Input: part model. Units: mm. Frame: model coordinates. A direction names the side the tool comes from. Give positions to 0.01 mm unless a question says otherwise; leave off trailing zeros. Loops run counter-clockwise (first coordinate to the right, second up) from the corner with the lowest first, then second, coordinate; pieces in that order, holes last. Notation, with made-up numbers: M 80.5,0 L 110.5,0 A11 cw 110.5,17 Z; hole C -34.5,86.25 d8. An arc over 180 degrees is marked long. Use CSV: the item, a comma, the result in double quotes. Start each with the question number.
Q1. Section A-A, the plane x = -2. Output: boundary loops of the cut face in (y, z).
Q2. Reachability of faces 1 (the flat face through (-3, 39, 0)), 2 (the flat face through (3, 39, 0)), 3 (the flat face through (0, 39, 3)), 4 (the flat face through (0, 39, -3)) from +Z, -Z, +X, -X, +Y, -Y: full face, straight path, thin tool, end or side. Return the list, or none.
Q3. Material intervals for line 1 along Y through (x, z) = (8.25, 0.5); line 2 along X through (y, z) = (74, 1), sorted ascending.
Q4. Section D-D, the plane x = -6.5. Output: boundary loops of the cut face in (y, z).
Q5. Section B-B, the plane z = -0.5. Output: boundary loops of the cut face in (x, y).
Q6. Pin query (flat end, axial travel): pin 1 (1.8 mm diameter, centred on x = 0.5, y = 47, fed in from -Z); pin 2 (1.8 mm diameter, centred on x = 0.5, y = 60, fed in from +Z); pin 3 (3 mm diameter, centred on y = 20, z = 0.5, fed in from +X); pin 4 (5 mm diameter, centred on y = 21.5, z = -7, fed in from +X). Return the tip coordinate at first contact, or that it passes through.
Q7. Section C-C, the plane y = 57. Output: boundary loops of the cut face in (x, z).
from build123d import *

# Parameters (mm, degrees)
SKETCH1_W           = 6
SKETCH1_H           = 6
BOSS_EXTRUDE1_DEPTH = 100
SKETCH2_W           = 20
SKETCH2_H           = 20
BOSS_EXTRUDE2_DEPTH = 20


with BuildPart() as part:
    # Sketch1 → Boss-Extrude1 (new body)
    with BuildSketch(Plane(origin=(0, 0, 0), x_dir=(1, 0, 0), z_dir=(0, 1, 0))):
        Rectangle(SKETCH1_W, SKETCH1_H)
    extrude(amount=BOSS_EXTRUDE1_DEPTH)

    # Sketch2 → Boss-Extrude2 (add)
    with BuildSketch(Plane(origin=(0, 100, 0), x_dir=(1, 0, 0), z_dir=(0, 1, 0))):
        Rectangle(SKETCH2_W, SKETCH2_H)
    extrude(amount=-BOSS_EXTRUDE2_DEPTH)


solid = part.part
A:
1,outline,"M 0,-3 L 80,-3 L 80,-10 L 100,-10 L 100,10 L 80,10 L 80,3 L 0,3 Z"
2,face 1,"+Z, -Z, -X, -Y"
2,face 2,"+Z, -Z, +X, -Y"
2,face 3,"+Z, +X, -X, -Y"
2,face 4,"-Z, +X, -X, -Y"
3,line 1,"80 to 100"
3,line 2,"-3 to 3"
4,outline,"M 80,-10 L 100,-10 L 100,10 L 80,10 Z"
5,outline,"M -10,80 L -3,80 L -3,0 L 3,0 L 3,80 L 10,80 L 10,100 L -10,100 Z"
6,pin 1,"z = -3"
6,pin 2,"z = 3"
6,pin 3,"x = 3"
6,pin 4,"through"
7,outline,"M -3,-3 L 3,-3 L 3,3 L -3,3 Z"
